```python
from build123d import *

# Parameters (mm, degrees)
BOSS_EXTRUDE1_DEPTH = 2.55
SKETCH5_OUTSIDE_W   = 43.682
SKETCH5_OUTSIDE_H   = 44.92
SKETCH5_OUTSIDE_R   = 4
CUT_EXTRUDE1_DEPTH  = 8.958852514
CUT_EXTRUDE1_DRAFT  = -60
SKETCH6_OUTSIDE_W   = 43.682
SKETCH6_OUTSIDE_H   = 44.92
SKETCH6_OUTSIDE_R   = 4
CUT_EXTRUDE2_DEPTH  = 8.958852514
CUT_EXTRUDE2_DRAFT  = -60
CUT_EXTRUDE3_DEPTH  = 0.635


with BuildPart() as part:
    # Sketch4 → Boss-Extrude1 (new, symmetric)
    with BuildSketch(Plane.XY):
        Polygon((-4, 2.309401077), (-4, -2.309401077), (0, -4.618802154), (4, -2.309401077), (4, 2.309401077), (0, 4.618802154), align=None)
    extrude(amount=BOSS_EXTRUDE1_DEPTH, both=True)


with BuildPart() as cut_extrude1_tool:
    # Sketch5 outside → Cut-Extrude1 (with draft: the straight prism first)
    with BuildSketch(Plane.XY.offset(2.55)):
        Rectangle(SKETCH5_OUTSIDE_W, SKETCH5_OUTSIDE_H)
        Circle(SKETCH5_OUTSIDE_R, mode=Mode.SUBTRACT)
    extrude(amount=-CUT_EXTRUDE1_DEPTH)
    # Cut-Extrude1: the draft: its side faces are tilted about the plane it starts from
    cut_extrude1_sides = [cut_extrude1_tool.faces().sort_by_distance(p)[0] for p in [
        (0, -22.46, -1.929426257),
        (21.841, 0, -1.929426257),
        (0, 22.46, -1.929426257),
        (-21.841, 0, -1.929426257),
        (-4, 0, -1.929426257),
    ]]
    draft(cut_extrude1_sides, Plane.XY.offset(2.55), CUT_EXTRUDE1_DRAFT)


with BuildPart() as part_1:
    add(part.part)

    # Cut-Extrude1: cut by cut_extrude1_tool
    add(cut_extrude1_tool.part, mode=Mode.SUBTRACT)


with BuildPart() as cut_extrude2_tool:
    # Sketch6 outside → Cut-Extrude2 (with draft: the straight prism first)
    with BuildSketch(Plane(origin=(0, 0, -2.55), x_dir=(-1, 0, 0), z_dir=(0, 0, -1))):
        Rectangle(SKETCH6_OUTSIDE_W, SKETCH6_OUTSIDE_H)
        Circle(SKETCH6_OUTSIDE_R, mode=Mode.SUBTRACT)
    extrude(amount=-CUT_EXTRUDE2_DEPTH)
    # Cut-Extrude2: the draft: its side faces are tilted about the plane it starts from
    cut_extrude2_sides = [cut_extrude2_tool.faces().sort_by_distance(p)[0] for p in [
        (0, -22.46, 1.929426257),
        (-21.841, 0, 1.929426257),
        (0, 22.46, 1.929426257),
        (21.841, 0, 1.929426257),
        (4, 0, 1.929426257),
    ]]
    draft(cut_extrude2_sides, Plane(origin=(0, 0, -2.55), x_dir=(-1, 0, 0), z_dir=(0, 0, -1)), CUT_EXTRUDE2_DRAFT)


with BuildPart() as part_2:
    add(part_1.part)

    # Cut-Extrude2: cut by cut_extrude2_tool
    add(cut_extrude2_tool.part, mode=Mode.SUBTRACT)

    # Sketch7 → Cut-Revolve1 (revolve, cut)
    with BuildSketch(Plane(origin=(0, 0, 0), x_dir=(0, 0, -1), z_dir=(1, 0, 0))):
        Polygon((2.55, 0), (-2.55, 0), (-2.55, 2.58660254), (-2.46339746, 2.5), (2.46339746, 2.5), (2.55, 2.58660254), align=None)
    revolve(axis=Axis((0, 0, -2.55), (0, 0, 1)), mode=Mode.SUBTRACT)

    # Sketch8 → Cut-Extrude3 (cut)
    with BuildSketch(Plane.XY.offset(2.55)):
        Polygon((-2.65010254, 0), (-4, -0.779363662), (-4, 0.779363662), align=None)
        Polygon((4, -0.779363662), (4, 0.779363662), (2.65010254, 0), align=None)
    extrude(amount=-CUT_EXTRUDE3_DEPTH, mode=Mode.SUBTRACT)


solid = part_2.part
```
For this review, take the finished solid that the model builds, in its own axes (mm). A direction names the side the tool comes from. Give positions to 0.01 mm unless a question says otherwise; leave off trailing zeros. Write each loop counter-clockwise with the first axis right and the second up, starting at its lowest first coordinate (ties: lowest second). Pieces come first, ordered by that corner, then holes. Notation, with made-up numbers: M 11.5,2 L 40.5,2 A19 ccw 40.5,18 Z; hole C 2,4.25 d10. An arc over 180 degrees is marked long. Answer as a JSON object with one key per item and string values. Group by question number.
Item 1: Tool access review of faces 1 (the conical face through (-3.602, 2.096, 2.453)), 2 (the flat face through (3, 0, 1.915)): name each direction out of +Z, -Z, +X, -X, +Y, -Y from which nothing blocks a thin tool from reaching the whole face with its end or side.
Item 2: Draft analysis for pull direction Y (two halves, no side actions). For faces 3 (the cylindrical face through (2.44, -0.54, -0.03)), 4 (the conical face through (0.01, 4.148, 2.465)), 5 (the conical face through (3.602, -2.096, 2.453)), 6 (the flat face through (-3, 0, 1.915)), state which applies: +Y half, -Y half, draft (parallel to the pull), parting line (faces both ways), or undercut.
Item 3: For pin 1 Ø1.5 at (x, z) = (2.5, 0.5) entering from +Y; pin 2 Ø1 at (x, z) = (1, 2) entering from -Y, all flat-tipped, find the tip position at first contact; note any pin that passes through.
Item 4: Consider section A-A on z = 0.5. Write out the cut boundary in (x, y), plus the area to 3 significant figures.
Item 5: For probe 1 along X at (y, z) = (0, 0.8); probe 2 along X at (y, z) = (0.5, -2.1); probe 3 along Y at (x, z) = (3.25, 2.15), list the stretches that pass through material, from the lowest coordinate up. Write a range as [from, to].
Check result:
{
 "1": {"face 1": "+Z, -X, +Y", "face 2": "+Z, +X"},
 "2": {"face 3": "undercut", "face 4": "+Y half", "face 5": "-Y half", "face 6": "undercut"},
 "3": {"pin 1": "stops at y = 3.61", "pin 2": "stops at y = -4.33"},
 "4": {"outline": "M -4,-2.31 L 0,-4.62 L 4,-2.31 L 4,2.31 L 0,4.62 L -4,2.31 Z; hole C 0,0 d5", "area": "35.8 mm^2"},
 "5": {"probe 1": "x = [-4, -2.5], [2.5, 4]", "probe 2": "x = [-4, -2.45], [2.45, 4]", "probe 3": "y = [-2.74, -0.35], [0.35, 2.74]"}
}
